Autodesk Inventor part; units mm, degrees
ref_plane "Arbeitsebene1" through (20, 0, 0) normal (1, 0, 0) x (0, 1, 0)
ref_plane "XZ Plane" through (0, 0, 0) normal (0, 1, 0) x (-1, 0, 0)
ref_plane "XY Plane" through (0, 0, 0) normal (0, 0, 1) x (1, 0, 0)
sketch "Skizze3" plane through (0, 0, 0) normal (0, 1, 0) x (-1, 0, 0)
  point P0 (0, 0)
sketch "Skizze4" plane through (0, 0, 0) normal (0, 0, 1) x (1, 0, 0)
  line L0 (0, 0) -> (20, 0)
  line L1 (20, 0) -> (20, 10)
  line L2 (20, 10) -> (40, 25)
  line L3 (40, 25) -> (40, 30)
  line L4 (40, 30) -> (0, 30)
  line L5 (0, 30) -> (0, 0)
  dimension "d5" = 40
  dimension "d6" = 80
  dimension "d7" = 10
  dimension "d8" = 15
  dimension "d9" = 5
revolve "Umdrehung1" add sketch "Skizze4" angle 360 about axis through (0, 30, 0) along (0, -1, 0)
sketch "Skizze5" plane through (0, 30, 0) normal (0, 1, 0) x (1, 0, 0)
  circle A0 centre (0, -25) radius 2.5
  line L0 (0, 56) -> (0, -56)
  point P0 (0, 0)
  dimension "d11" = 25
  dimension "d12" = 5
extrude "Extrusion3" cut sketch "Skizze5" against normal blind 12.1
chamfer "Fase1" distance 0.5 angle 45 1 edges at (-2.5, 30, 25)
pattern_circular "Runde Anordnung1" count 6 over 360 about axis through (0, 5, 0) along (0, -1, 0) of "Extrusion3", "Fase1"
ref_plane "Arbeitsebene1" through (20, 0, 0) normal (1, 0, 0) x (0, 1, 0)
sketch "Skizze6" plane through (20, 0, 0) normal (1, 0, 0) x (0, 1, 0)
  line L0 (10, 20) -> (10, -20)
  line L1 (0, 20) -> (0, -20)
  line L2 (-2.9204, 0) -> (2.9204, 0)
  point P0 (0, 0)
  point P1 (5, 0)
  point P2 (0, 0)
  dimension "d22" = 5
sketch "Skizze7" plane through (0, 0, 0) normal (0, -1, 0) x (1, 0, 0)
  circle A0 centre (0, 0) radius 3
  line L0 (1.199, 2.75) -> (1.199, -2.75)
  point P0 (0, 0)
  dimension "d23" = 6
  dimension "d24" = 5.5
extrude "Extrusion4" cut sketch "Skizze7" against normal blind 12.2 contours L0 A0 picked at (-0.2225, -0.8366)
hole "Bohrung1" at (20, 5, 0) direction (-1, 0, 0) diameter 4.134 depth 18.801
chamfer "Fase2" distance 0.5 angle 45 3 edges at (19.8929, 4.9998, 2.067) (19.9385, 6.3471, -1.5678) (19.9383, 3.6548, -1.5694)
properties part number "BT405_trajan20_21" material "Kunststoff, undurchsichtig Schwarz"
CAD build for the part. Positions are in the model's coordinates, mm. A direction names the side the tool comes from. Coordinates: 2 decimals unless noted, no trailing zeros. Order: outer loops, then holes, each group sorted by start corner. A loop starts at its lowest first (then second) coordinate and runs counter-clockwise, first axis right, second up. Notation, with made-up numbers: (-11.5, 22.5) -> (18.5, 22.5) arc R16 cw to (18.5, 39.5) -> close; hole circle Ø8 at (8, 70). An arc over 180 degrees is marked (long way). Answer in a Markdown table with one row per item.
1) Mould opens along Z. For faces 1 (the face through (-4.61, 10.94, 20.75)), 2 (the face through (-22, 17.9, -13)), 3 (the face through (4, 0, 0)) say: pulls with the +Z half, pulls with the -Z half, needs draft (parallel to the pull), parting line crosses it, or undercut.
Check values:
| item | result |
|---|---|
| face 1 | parting line crosses it |
| face 2 | undercut |
| face 3 | needs draft |
2) Flat gauge pins, fed straight in: P1, Ø8, axis at x = 26.5, z = -12.5, coming from the -Y side; P2, Ø6, axis at x = 21.65, z = -12.5, coming from the -Y side; P3, Ø4.5, axis at x = 21.65, z = 12.5, coming from the -Y side. Where does each tip first touch, or does it go through?
Check values:
| item | result |
|---|---|
| P1 | y = 13.98 |
| P2 | y = 11.5 |
| P3 | y = 12.06 |
3) Which spindle directions (+Z, -Z, +X, -X, +Y, -Y) get a long thin tool onto all of the face, cutting with end or side? Do faces 4 (the face through (10.22, 2.95, 0.27)), 5 (the face through (-3, 6, 0)), 6 (the face through (22, 17.9, 13)). Say none if no direction does.
Check values:
| item | result |
|---|---|
| face 4 | +X |
| face 5 | -Y |
| face 6 | +Y |
4) Band-saw the part on A-A (x = 0). List the corners of the cut face in (y, z).
Check values:
| item | result |
|---|---|
| outline | (0, -20) -> (10, -20) -> (25, -40) -> (30, -40) -> (30, -28) -> (29.5, -27.5) -> (17.9, -27.5) -> (17.9, -22.5) -> (29.5, -22.5) -> (30, -22) -> (30, 22) -> (29.5, 22.5) -> (17.9, 22.5) -> (17.9, 27.5) -> (29.5, 27.5) -> (30, 28) -> (30, 40) -> (25, 40) -> (10, 20) -> (0, 20) -> (0, 3) -> (12.2, 3) -> (12.2, -3) -> (0, -3) -> close |
5) Drill centre lines: line 1 (Y direction, x = 12, z = 0); line 2 (Z direction, x = -23.5, y = 25.5); line 3 (X direction, y = 21, z = 25). Where is each one in solid material? Low to high.
Check values:
| item | result |
|---|---|
| line 1 | 0 to 2.93, 7.07 to 30 |
| line 2 | -32.37 to -14.18, -10.82 to 10.82, 14.18 to 32.37 |
| line 3 | -24.02 to -2.5, 2.5 to 24.02 |
